from build123d import *

# Parameters (mm, degrees)
SKETCH1_R                  = 0.5
SKETCH1_W                  = 46.5
SKETCH1_H                  = 16
SKETCH1_W_2                = 16
SKETCH1_H_2                = 46.5
BOSS_EXTRUDE1_DEPTH        = 1.6
F_3_2_3_2_DIAMETER_HOLE3_D = 3.2
FILLET1_R                  = 3
FILLET2_R                  = 1


with BuildPart() as part:
    # Sketch1 → Boss-Extrude1 (new body)
    with BuildSketch(Plane.XY):
        with BuildLine():
            Line((-87.56534388, 88.95185693), (-87.56534388, 6.95185693))
            ThreePointArc((-87.56534388, 6.95185693), (-86.686664224, 4.830536587), (-84.56534388, 3.95185693))
            Line((-84.56534388, 3.95185693), (-71.56534388, 3.95185693))
            Line((-71.56534388, 3.95185693), (-71.56534388, 9.95185693))
            Line((-71.56534388, 9.95185693), (-55.56534388, 9.95185693))
            Line((-55.56534388, 9.95185693), (-55.56534388, 3.95185693))
            Line((-55.56534388, 3.95185693), (3.43465612, 3.95185693))
            ThreePointArc((3.43465612, 3.95185693), (5.555976464, 4.830536587), (6.43465612, 6.95185693))
            Line((6.43465612, 6.95185693), (6.43465612, 88.95185693))
            ThreePointArc((6.43465612, 88.95185693), (5.555976464, 91.073177274), (3.43465612, 91.95185693))
            Line((3.43465612, 91.95185693), (-33.06534388, 91.95185693))
            Line((-33.06534388, 91.95185693), (-33.06534388, 85.95185693))
            Line((-33.06534388, 85.95185693), (-48.06534388, 85.95185693))
            Line((-48.06534388, 85.95185693), (-48.06534388, 91.95185693))
            Line((-48.06534388, 91.95185693), (-84.56534388, 91.95185693))
            ThreePointArc((-84.56534388, 91.95185693), (-86.686664224, 91.073177274), (-87.56534388, 88.95185693))
        make_face()
        with Locations((-63.52534388, 18.55185693)):
            Circle(SKETCH1_R, mode=Mode.SUBTRACT)
        with Locations((-68.60534388, 18.55185693)):
            Circle(SKETCH1_R, mode=Mode.SUBTRACT)
        with Locations((-29.81534388, 21.45185693)):
            Rectangle(SKETCH1_W, SKETCH1_H, mode=Mode.SUBTRACT)
        with Locations((-62.56534388, 56.70185693)):
            Rectangle(SKETCH1_W_2, SKETCH1_H_2, mode=Mode.SUBTRACT)
    extrude(amount=BOSS_EXTRUDE1_DEPTH)

    # Ø3.2 (3.2) Diameter Hole3 (through all)
    with Locations(Plane(origin=(0, 0, 0), x_dir=(-1, 0, 0), z_dir=(0, 0, -1))):
        with Locations((78.56534388, 6.95185693), (78.56534388, 82.95185693), (2.56534388, 82.95185693), (2.56534388, 6.95185693), (2.56534388, 65.45185693), (2.56534388, 20.45185693), (62.56534388, 82.95185693), (48.56534388, 6.95185693), (28.06534388, 88.95185693), (61.31534388, 88.95185693), (-2.93465612, 56.618523597), (-2.93465612, 33.285190263), (23.81534388, 6.95185693)):
            Hole(F_3_2_3_2_DIAMETER_HOLE3_D / 2)

    # Fillet1
    fillet1_edges = [part.edges().sort_by_distance(p)[0] for p in [
        (-48.06534388, 85.95185693, 0.8),
        (-33.06534388, 85.95185693, 0.8),
        (-55.56534388, 9.95185693, 0.8),
        (-71.56534388, 9.95185693, 0.8),
    ]]
    fillet(fillet1_edges, radius=FILLET1_R)

    # Fillet2
    fillet2_edges = [part.edges().sort_by_distance(p)[0] for p in [
        (-48.06534388, 91.95185693, 0.8),
        (-33.06534388, 91.95185693, 0.8),
        (-55.56534388, 3.95185693, 0.8),
        (-71.56534388, 3.95185693, 0.8),
        (-6.56534388, 13.45185693, 0.8),
        (-6.56534388, 29.45185693, 0.8),
        (-53.06534388, 29.45185693, 0.8),
        (-53.06534388, 13.45185693, 0.8),
        (-54.56534388, 33.45185693, 0.8),
        (-54.56534388, 79.95185693, 0.8),
        (-70.56534388, 79.95185693, 0.8),
        (-70.56534388, 33.45185693, 0.8),
    ]]
    fillet(fillet2_edges, radius=FILLET2_R)


solid = part.part
Could you check a few things on this model? Use its own coordinates, in mm. A direction names the side the tool comes from. Give positions to 0.01 mm unless a question says otherwise; leave off trailing zeros. Order: outer loops, then holes, each group sorted by start corner. A loop starts at its lowest first (then second) coordinate and runs counter-clockwise, first axis right, second up.
1. Suppose I cut it at B-B (x = -10.5). Write out the boundary of the cut face in (y, z).
Answers below:
outline: (3.95, 0) - (13.45, 0) - (13.45, 1.6) - (3.95, 1.6) - close; (29.45, 0) - (91.95, 0) - (91.95, 1.6) - (29.45, 1.6) - close
2. Suppose I cut it at A-A (y = 53.5). Write out the boundary of the cut face in (x, z).
Answers below:
outline: (-87.57, 0) - (-70.57, 0) - (-70.57, 1.6) - (-87.57, 1.6) - close; (-54.57, 0) - (6.43, 0) - (6.43, 1.6) - (-54.57, 1.6) - close
3. Suppose I cut it at C-C (z = 0.3). State how many separate pieces and enclosed holes the cut face has, plus the area to 3 significant figures.
Answers below:
separate pieces: 1
enclosed holes: 17
area: 6,490 mm2
4. Which directions (+Z, -Z, +X, -X, +Y, -Y) give clear straight access to the entire face, cutting with the end or side of a thin tool? Please do faces 1 (the cylindrical face through (-47.21, 86.854, 0.811)), 2 (the cylindrical face through (-86.71, 4.854, 0.789)), 3 (the cylindrical face through (-70.71, 9.05, 0.81)).
Answers below:
face 1: +Z, -Z, +Y
face 2: +Z, -Z, -X, -Y
face 3: +Z, -Z, -Y
5. I need wall thicknesses on L1, parallel to Y at x = -18, z = 0.1; L2, parallel to X at y = 71, z = 1.5; L3, parallel to Y at x = -2.5, z = 0.9. Which ranges of each line are inside material? Lowest first, please.
Answers below:
L1: y = 3.95 to 13.45, 29.45 to 91.95
L2: x = -87.57 to -70.57, -54.57 to 6.43
L3: y = 3.95 to 5.35, 8.55 to 18.85, 22.05 to 63.85, 67.05 to 81.35, 84.55 to 91.95
6. For pin 1 (0.8 mm diameter, centred on x = -61, z = 1, fed in from -Y); pin 2 (0.8 mm diameter, centred on x = -42, z = 0.5, fed in from +Y); pin 3 (0.8 mm diameter, centred on y = 6, z = 1, fed in from -X), each with a flat end and sliding along its axis, tell me the tip position at first contact or that it passes through.
Answers below:
pin 1: stops at y = 9.95
pin 2: stops at y = 85.95
pin 3: stops at x = -87.51
